```python
from build123d import *

# Parameters (mm, degrees)
CHAMFER1_SIZE = 0.25


with BuildPart() as part:
    # Sketch1 → Revolve2 (revolve)
    with BuildSketch(Plane.XY, mode=Mode.PRIVATE) as revolve2_sk:
        with BuildLine():
            Line((0, 0), (0, 6))
            Line((0, 6), (0, 7.5))
            Line((0, 7.5), (1.322875656, 7.5))
            ThreePointArc((1.322875656, 7.5), (1.822875656, 6.822875656), (2, 6))
            Line((2, 6), (1.5, 6))
            Line((1.5, 6), (1.5, 2))
            Line((1.5, 2), (1.15, 2))
            Line((1.15, 2), (1.15, 1.4))
            Line((1.15, 1.4), (1.5, 1.4))
            Line((1.5, 1.4), (1.5, 0))
            Line((1.5, 0), (0, 0))
        make_face()
    revolve(revolve2_sk.sketch.rotate(Axis((0, 0, 0), (0, 1, 0)), 90), axis=Axis((0, 0, 0), (0, 1, 0)))

    # Chamfer1
    chamfer1_edges = [part.edges().sort_by_distance(p)[0] for p in [
        (0, 0, 1.5),
    ]]
    chamfer(chamfer1_edges, length=CHAMFER1_SIZE)


solid = part.part
```
The listing builds one solid part. Answer for the finished solid, in the listing's coordinates (mm). A direction names the side the tool comes from. Round coordinates to 2 decimals unless told otherwise and drop trailing zeros. Write each loop counter-clockwise with the first axis right and the second up, starting at its lowest first coordinate (ties: lowest second). Pieces come first, ordered by that corner, then holes. Notation, with made-up numbers: (-22, 26.25) -> (25, 26.25) arc R24 ccw to (25, 55.25) -> close; hole circle Ø6 at (-14, 19). An arc over 180 degrees is marked (long way). Use CSV: the item, a comma, the result in double quotes. Start each with the question number.
(1) The mould has two halves that part along Y. Classify faces 3 (the face through (0, 7.5, 0)), 4 (the face through (0.7, 1.7, 0.91)), 5 (the face through (-0.45, 0.82, -1.43)): released by +Y, released by -Y, zero draft, split by the parting line, or undercut.
(2) Consider L1, parallel to X at y = 3.25, z = -0.05; L2, parallel to Y at x = -0.1, z = -1.45. Determine where each line is inside the solid, lowest interval first. Write a range as from..to.
(3) Section C-C on y = 1.25 is taken. Give the vertices of the cut face in (x, z), then the cut area to 3 significant figures.
(4) Which of the six approach directions +Z, -Z, +X, -X, +Y, -Y give full straight-line access (tool end or side, diameter ignored) to faces 1 (the face through (-0.45, 3.97, -1.43)), 2 (the face through (0, 0, 0))?
(5) This flat-tipped pin is pushed along its axis until it touches: pin 1 (2 mm diameter, centred on y = 2, z = 1.5, fed in from +X). Where does it stop, or does it pass through?
(6) Section B-B on z = 0 is taken. Give the vertices of the cut face in (x, y), then the cut area to 3 significant figures.
(7) Section A-A on x = 0 is taken. Give the vertices of the cut face in (y, z).
(8) Section D-D on y = 6.5 is taken. Give the vertices of the cut face in (x, z), then the cut area to 3 significant figures.
A:
1,face 3,"released by +Y"
1,face 4,"undercut"
1,face 5,"zero draft"
2,L1,"x = -1.5..1.5"
2,L2,"y = 0.2..1.4, 2..7.37"
3,outline,"circle Ø3 at (0, 0)"
3,area,"7.07 mm²"
4,face 1,"-Y"
4,face 2,"+Z, -Z, +X, -X, -Y"
5,pin 1,"stops at x = 1.41"
6,outline,"(-2, 6) -> (-1.5, 6) -> (-1.5, 2) -> (-1.15, 2) -> (-1.15, 1.4) -> (-1.5, 1.4) -> (-1.5, 0.25) -> (-1.25, 0) -> (1.25, 0) -> (1.5, 0.25) -> (1.5, 1.4) -> (1.15, 1.4) -> (1.15, 2) -> (1.5, 2) -> (1.5, 6) -> (2, 6) arc R2 ccw to (1.32, 7.5) -> (-1.32, 7.5) arc R2 ccw to start"
6,area,"22.9 mm²"
7,outline,"(0, -1.25) -> (0.25, -1.5) -> (1.4, -1.5) -> (1.4, -1.15) -> (2, -1.15) -> (2, -1.5) -> (6, -1.5) -> (6, -2) arc R2 ccw to (7.5, -1.32) -> (7.5, 1.32) arc R2 ccw to (6, 2) -> (6, 1.5) -> (2, 1.5) -> (2, 1.15) -> (1.4, 1.15) -> (1.4, 1.5) -> (0.25, 1.5) -> (0, 1.25) -> close"
8,outline,"circle Ø3.87 at (0, 0)"
8,area,"11.8 mm²"
